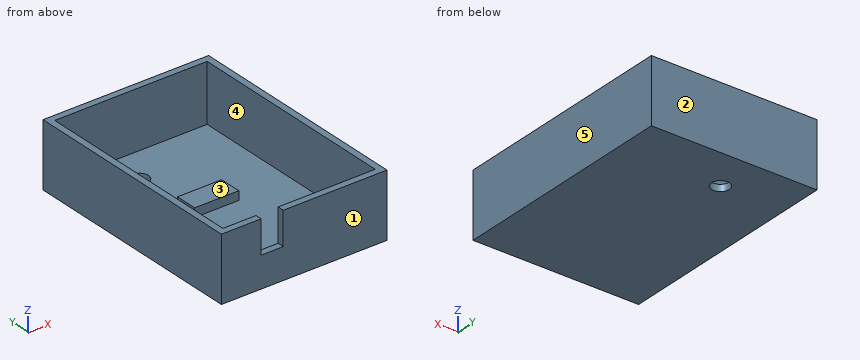
```python
from build123d import *

# Parameters (mm, degrees)
F0_W     = 37.5
F0_H     = 52
F1_DEPTH = 14.5
F2_W     = 34.5
F2_H     = 49
F3_DEPTH = 13
F4_R     = 2
F5_DEPTH = 25
F6_W     = 10
F6_H     = 5
F7_DEPTH = 2
F8_W     = 5
F8_H     = 7.5
F9_DEPTH = 10


with BuildPart() as f1:
    # F0 (on Top) → F1 (new body)
    with BuildSketch(Plane.XY):
        Rectangle(F0_W, F0_H)
    extrude(amount=F1_DEPTH)

    # F2 (on face) → F3 (cut)
    with BuildSketch(Plane.XY.offset(14.5)):
        Rectangle(F2_W, F2_H)
    extrude(amount=-F3_DEPTH, mode=Mode.SUBTRACT)

    # F4 (on face) → F5 (cut)
    with BuildSketch(Plane.XY.offset(1.5)):
        with Locations((-4.25, 16.5)):
            Circle(F4_R)
    extrude(amount=-F5_DEPTH, mode=Mode.SUBTRACT)

    # F6 (on face) → F7 (join)
    with BuildSketch(Plane.XY.offset(1.5)):
        with Locations((0, 2)):
            Rectangle(F6_W, F6_H)
    extrude(amount=F7_DEPTH)

    # F8 (on face) → F9 (cut)
    with BuildSketch(Plane.XZ.offset(26)):
        with Locations((-7.25, 10.75)):
            Rectangle(F8_W, F8_H)
    extrude(amount=-F9_DEPTH, mode=Mode.SUBTRACT)


solid = f1.part
```
For this review, take the finished solid that the model builds, in its own axes (mm). Face numbers are marked on the shaded views. A direction names the side the tool comes from. Round coordinates to 2 decimals unless told otherwise and drop trailing zeros. Write each loop counter-clockwise with the first axis right and the second up, starting at its lowest first coordinate (ties: lowest second). Pieces come first, ordered by that corner, then holes. Notation, with made-up numbers: (45, 10) -> (70, 10) arc R24 ccw to (70, 38) -> close; hole circle Ø5 at (-5.5, 78). An arc over 180 degrees is marked (long way). One line per question, with ' | ' between items. Start each with the question number.
1) Add section C-C (x = 7.5). Write out the cut boundary in (y, z), and give its area (3 significant figures).
2) Add section D-D (y = -4). Write out the cut boundary in (x, z).
3) Machinability: for the marked faces 4 and 5, which of the approach directions +Z, -Z, +X, -X, +Y, -Y give a long, thin tool a straight path to every point of the face, cutting with its end or side? Answer none if there is none.
4) Mouldability with a two-part tool opening along Y and no side actions: class the marked faces 1, 2 and 3 as +Y half, -Y half, draft (parallel to the pull), parting line (faces both ways), or undercut.
5) Add section B-B (z = 5.75). Write out the cut boundary in (x, y), and give its area (4 significant figures).
6) Wall thickness on line 1 along X through (y, z) = (4, 2.5); line 2 along Y through (x, z) = (1.5, 1.75); line 3 along X through (y, z) = (-10, 6.5): over which ranges is each line inside the solid? List them lowest first.
7) For pin 1 Ø3.5 at (x, y) = (-4.25, 16.5) entering from -Z; pin 2 Ø10 at (x, y) = (-6.5, 18.5) entering from +Z; pin 3 Ø1.5 at (x, y) = (-0.5, 1) entering from +Z; pin 4 Ø0.8 at (x, y) = (-8.5, -25.5) entering from +Z, all flat-tipped, find the tip position at first contact; note any pin that passes through.
8) Add section A-A (y = 16.5). Write out the cut boundary in (x, z), and give its area (4 significant figures).
Reported:
1) outline: (-26, 0) -> (26, 0) -> (26, 14.5) -> (24.5, 14.5) -> (24.5, 1.5) -> (-24.5, 1.5) -> (-24.5, 14.5) -> (-26, 14.5) -> close | area: 117 mm²
2) outline: (-18.75, 0) -> (18.75, 0) -> (18.75, 14.5) -> (17.25, 14.5) -> (17.25, 1.5) -> (-17.25, 1.5) -> (-17.25, 14.5) -> (-18.75, 14.5) -> close
3) face 4: +Z | face 5: +Z, -Z, +X, +Y, -Y
4) face 1: -Y half | face 2: +Y half | face 3: undercut
5) outline: (-18.75, -26) -> (18.75, -26) -> (18.75, 26) -> (-18.75, 26) -> close; hole (-17.25, -24.5) -> (17.25, -24.5) -> (17.25, 24.5) -> (-17.25, 24.5) -> close | area: 259.5 mm²
6) line 1: x = -18.75 to -17.25, -5 to 5, 17.25 to 18.75 | line 2: y = -26 to -24.5, -0.5 to 4.5, 24.5 to 26 | line 3: x = -18.75 to -17.25, 17.25 to 18.75
7) pin 1: passes through | pin 2: stops at z = 1.5 | pin 3: stops at z = 3.5 | pin 4: stops at z = 7
8) outline: (-18.75, 0) -> (-6.25, 0) -> (-6.25, 1.5) -> (-17.25, 1.5) -> (-17.25, 14.5) -> (-18.75, 14.5) -> close; (-2.25, 0) -> (18.75, 0) -> (18.75, 14.5) -> (17.25, 14.5) -> (17.25, 1.5) -> (-2.25, 1.5) -> close | area: 89.25 mm²
